The listing builds one solid part. Answer for the finished solid, in the listing's coordinates (mm). A direction names the side the tool comes from. Give positions to 0.01 mm unless a question says otherwise; leave off trailing zeros. Order: outer loops, then holes, each group sorted by start corner. A loop starts at its lowest first (then second) coordinate and runs counter-clockwise, first axis right, second up. Notation, with made-up numbers: (34, 84) -> (76, 84) arc R20 cw to (76, 96) -> close; hole circle Ø5 at (85.5, 28). An arc over 180 degrees is marked (long way). Answer as a JSON object with one key per item and string values. Group by question number.
```python
from build123d import *

# Parameters (mm, degrees)
F0_R     = 1.8
F0_R_2   = 3.435534
F1_DEPTH = 8
F2_DEPTH = 3
F3_R     = 1.8
F4_DEPTH = 2.4
F5_SIZE  = 1


with BuildPart() as f1:
    # F0 (on Top) → F1 (new body)
    with BuildSketch(Plane.XY):
        Polygon((34.5, 5.5), (-5.5, 5.5), (-5.5, -34.5), (2.5, -34.5), (2.5, -2.5), (34.5, -2.5), align=None)
        with Locations((-0.1, -27.5)):
            Circle(F0_R, mode=Mode.SUBTRACT)
        Circle(F0_R_2, mode=Mode.SUBTRACT)
        with Locations((27.5, 0.1)):
            Circle(F0_R, mode=Mode.SUBTRACT)
    extrude(amount=F1_DEPTH)

    # F0 (on Top) → F2 (join)
    with BuildSketch(Plane.XY):
        Polygon((2.5, -34.5), (34.5, -2.5), (2.5, -2.5), align=None)
        Circle(F0_R_2)
        Circle(F0_R, mode=Mode.SUBTRACT)
    extrude(amount=F2_DEPTH)

    # F3 (on face) → F4 (cut)
    with BuildSketch(Plane(origin=(0, 0, 0), x_dir=(1, 0, 0), z_dir=(0, 0, -1))):
        Polygon((-1.644435, 24.59402), (1.644435, 24.70949), (3.18887, 27.61547), (1.444435, 30.40598), (-1.844435, 30.29051), (-3.38887, 27.38453), align=None)
        with Locations((-0.1, 27.5)):
            Circle(F3_R, mode=Mode.SUBTRACT)
        Polygon((24.65, 1.545448), (24.65, -1.745448), (27.5, -3.390897), (30.35, -1.745448), (30.35, 1.545448), (27.5, 3.190897), align=None)
        with Locations((27.5, -0.1)):
            Circle(F3_R, mode=Mode.SUBTRACT)
    extrude(amount=-F4_DEPTH, mode=Mode.SUBTRACT)

    # F5
    f5_edges = [f1.edges().sort_by_distance(p)[0] for p in [
        (-5.5, 5.5, 4),
        (-5.5, -34.5, 4),
        (34.5, 5.5, 4),
        (14.5, 5.5, 8),
        (-5.5, -14.5, 8),
        (-1.5, -34.5, 8),
        (34.5, 1.5, 8),
    ]]
    chamfer(f5_edges, length=F5_SIZE)


solid = f1.part
```
(1) For a pull along Y with two mould halves and no side action, classify faces 1 (the flat face through (28.94, -2.36, 1.18)), 2 (the flat face through (-1, -34, 7.5)), 3 (the flat face through (34, 1, 7.5)) as +Y half, -Y half, draft (parallel to the pull), parting line (faces both ways), or undercut.
(2) A cutting plane is placed at A-A (z = 5). Determine the outline of the cut face in (x, y).
(3) A cutting plane is placed at D-D (x = 23). Determine the outline of the cut face in (y, z), and give its area (3 significant figures).
(4) Which of the six approach directions +Z, -Z, +X, -X, +Y, -Y give full straight-line access (tool end or side, diameter ignored) to faces 4 (the flat face through (-2.606, -28.858, 1.183)), 5 (the flat face through (-5, -34, 3)), 6 (the flat face through (18, -2.5, 5))?
(5) A cutting plane is placed at B-B (y = -1). Determine the outline of the cut face in (x, z), and give its area (3 significant figures).
(6) A cutting plane is placed at C-C (x = 0). Determine the outline of the cut face in (y, z), and give its area (3 significant figures).
(7) Find the intervals of material crossed by line 1 along Y through (x, z) = (0, 5.45); line 2 along X through (y, z) = (0.1, 5.8); line 3 along Y through (x, z) = (0.5, 0.75), in increasing order. Write a range as [from, to].
(8) Flat-ended cylindrical pins translate along their axes: pin 1 Ø4 at (y, z) = (-18.5, 4.5) entering from +X; pin 2 Ø2.5 at (x, z) = (19, 4.5) entering from -Y; pin 3 Ø3 at (x, y) = (1, -27) entering from -Z. Find the tip coordinate at first contact, or state that the pin passes through.
Check sheet entries:
{
 "1": {"face 1": "undercut", "face 2": "-Y half", "face 3": "draft"},
 "2": {"outline": "(-5.5, -33.5) -> (-4.5, -34.5) -> (2.5, -34.5) -> (2.5, -2.5) -> (34.5, -2.5) -> (34.5, 4.5) -> (33.5, 5.5) -> (-4.5, 5.5) -> (-5.5, 4.5) -> close; hole circle Ø6.87 at (0, 0); hole circle Ø3.6 at (-0.1, -27.5); hole circle Ø3.6 at (27.5, 0.1)"},
 "3": {"outline": "(-14, 0) -> (5.5, 0) -> (5.5, 7) -> (4.5, 8) -> (-2.5, 8) -> (-2.5, 3) -> (-14, 3) -> close", "area": "98.0 mm2"},
 "4": {"face 4": "-Z", "face 5": "+Z, -Z, -X, -Y", "face 6": "+Z, +X, -Y"},
 "5": {"outline": "(-5.5, 0) -> (-1.5, 0) -> (-1.5, 3) -> (-3.29, 3) -> (-3.29, 8) -> (-4.5, 8) -> (-5.5, 7) -> close; (1.5, 0) -> (24.65, 0) -> (24.65, 2.4) -> (26.08, 2.4) -> (26.08, 8) -> (3.29, 8) -> (3.29, 3) -> (1.5, 3) -> close; (28.92, 2.4) -> (30.35, 2.4) -> (30.35, 0) -> (34.5, 0) -> (34.5, 7) -> (33.5, 8) -> (28.92, 8) -> close", "area": "248 mm2"},
 "6": {"outline": "(-34.5, 0) -> (-30.36, 0) -> (-30.36, 2.4) -> (-29.3, 2.4) -> (-29.3, 8) -> (-33.5, 8) -> (-34.5, 7) -> close; (-25.7, 2.4) -> (-24.65, 2.4) -> (-24.65, 0) -> (-1.8, 0) -> (-1.8, 3) -> (-3.44, 3) -> (-3.44, 8) -> (-25.7, 8) -> close; (1.8, 0) -> (5.5, 0) -> (5.5, 7) -> (4.5, 8) -> (3.44, 8) -> (3.44, 3) -> (1.8, 3) -> close", "area": "240 mm2"},
 "7": {"line 1": "y = [-34.5, -29.3], [-25.7, -3.44], [3.44, 5.5]", "line 2": "x = [-5.5, -3.43], [3.43, 25.7], [29.3, 34.5]", "line 3": "y = [-34.5, -30.37], [-24.67, -1.73], [1.73, 5.5]"},
 "8": {"pin 1": "stops at x = 19.82", "pin 2": "stops at y = -2.5", "pin 3": "stops at z = 2.4"}
}
